Part model, mm, in its own coordinate system. A direction names the side the tool comes from. Round coordinates to 2 decimals unless told otherwise and drop trailing zeros. Write each loop counter-clockwise with the first axis right and the second up, starting at its lowest first coordinate (ties: lowest second). Pieces come first, ordered by that corner, then holes. Notation, with made-up numbers: M 81,-18 L 136,-18 A6 cw 136,-10 Z; hole C 22.5,3 d1. An arc over 180 degrees is marked long. Answer as a JSON object with one key per item and string values. Group by question number.
1. Drop flat-ended pins along their axis: pin 1 (2 mm diameter, centred on x = 13.4, z = 0, fed in from -Y); pin 2 (1.8 mm diameter, centred on x = -13, z = 1, fed in from +Y); pin 3 (3 mm diameter, centred on x = 0, z = 0, fed in from +Y); pin 4 (3 mm diameter, centred on x = 0, z = 0, fed in from -Y). Give the stop position or say it passes through.
2. Band-saw the part on C-C, the plane x = 1.5. Write the cut outline in (y, z).
3. Band-saw the part on B-B, the plane y = 3.55. Write the cut outline in (x, z).
4. Band-saw the part on A-A, the plane x = 9.8. Write the cut outline in (y, z), plus the area to 3 significant figures.
5. Drill centre lines: line 1 (X direction, y = 3.1, z = 0); line 2 (Y direction, x = 11.5, z = 1.25); line 3 (Z direction, x = 9.8, y = 0.5). Where is each one in solid material? Low to high. Write a range as from..to.
6. Two-plate mould, pull along Z, no slides. Class faces 1 (the face through (-8.628, 1.014, -2.473)), 2 (the face through (-5.15, 1.01, -0.03)), 3 (the face through (-8.75, 1.01, -0.03)), 4 (the face through (0, 0, -3)): +Z half, -Z half, draft (parallel to the pull), parting line (faces both ways), or undercut.
7. Which spindle directions (+Z, -Z, +X, -X, +Y, -Y) get a long thin tool onto all of the face, cutting with end or side? Do faces 5 (the face through (1, 1, 1)), 6 (the face through (1, 1.5, 1)), 7 (the face through (-12.685, 1.014, -0.225)). Say none if no direction does.
8. Band-saw the part on D-D, the plane x = 15.5. Write the cut outline in (y, z), plus the area to 3 significant figures.
from build123d import *

# Parameters (mm, degrees)
SKETCH1_W             = 3.5
SKETCH1_H             = 3.9
BOSS_EXTRUDE1_START   = -2
BOSS_EXTRUDE1_DEPTH   = 2
BOSS_EXTRUDE2_START   = -2
BOSS_EXTRUDE2_DEPTH   = 2
F_1_5MM_DOWEL_HOLE1_D = 1.5


with BuildPart() as part:
    # Sketch1 → Revolve1 (revolve)
    with BuildSketch(Plane.XY, mode=Mode.PRIVATE) as revolve1_sk:
        with Locations((1.75, 1.95)):
            Rectangle(SKETCH1_W, SKETCH1_H)
    revolve(revolve1_sk.sketch.rotate(Axis((0, 3.9, 0), (0, -1, 0)), 270), axis=Axis((0, 3.9, 0), (0, -1, 0)))

    # Sketch2 → Boss-Extrude1 (add)
    with BuildSketch(Plane.XZ.offset(BOSS_EXTRUDE1_START)):
        with BuildLine():
            Line((-1.868584713, 2.959457918), (-15.2, 2))
            ThreePointArc((-15.2, 2), (-17.2, 0), (-15.2, -2))
            Line((-15.2, -2), (-1.868584713, -2.959457918))
            ThreePointArc((-1.868584713, -2.959457918), (-3.5, 0), (-1.868584713, 2.959457918))
        make_face()
    extrude(amount=BOSS_EXTRUDE1_DEPTH)

    # Sketch3 → Boss-Extrude2 (add)
    with BuildSketch(Plane.XZ.offset(BOSS_EXTRUDE2_START)):
        with BuildLine():
            Line((1.868584713, -2.959457918), (15.2, -2))
            ThreePointArc((15.2, -2), (17.2, 0), (15.2, 2))
            Line((15.2, 2), (1.868584713, 2.959457918))
            ThreePointArc((1.868584713, 2.959457918), (3.5, 0), (1.868584713, -2.959457918))
        make_face()
    extrude(amount=BOSS_EXTRUDE2_DEPTH)

    # Sketch4 → Cut-Revolve1 (revolve, cut)
    with BuildSketch(Plane.XY, mode=Mode.PRIVATE) as cut_revolve1_sk:
        Polygon((2.45, 3.9), (0, 3.9), (0, 0), (2.35, 0), (2.35, 1), (1.2, 1), (1.2, 1.5), (2.45, 1.5), align=None)
    revolve(cut_revolve1_sk.sketch.rotate(Axis((0, 3.9, 0), (0, -1, 0)), 270), axis=Axis((0, 3.9, 0), (0, -1, 0)), mode=Mode.SUBTRACT)

    # Ø1.5mm Dowel Hole1 (through all)
    with Locations(Plane(origin=(0, 0, 0), x_dir=(-1, 0, 0), z_dir=(0, -1, 0))):
        with Locations((15.2, 0), (-15.2, 0), (13.4, 0), (11.6, 0), (9.8, 0), (8, 0), (6.2, 0), (4.4, 0), (-13.4, 0), (-11.6, 0), (-9.8, 0), (-8, 0), (-6.2, 0), (-4.4, 0)):
            Hole(F_1_5MM_DOWEL_HOLE1_D / 2)


solid = part.part
Worked answers:
{
 "1": {"pin 1": "stops at y = 0", "pin 2": "stops at y = 2", "pin 3": "stops at y = 1.5", "pin 4": "stops at y = 1"},
 "2": {"outline": "M 0,-3.16 L 3.9,-3.16 L 3.9,-1.94 L 1.5,-1.94 L 1.5,1.94 L 3.9,1.94 L 3.9,3.16 L 0,3.16 L 0,1.81 L 1,1.81 L 1,-1.81 L 0,-1.81 Z"},
 "3": {"outline": "C 0,0 d7; hole C 0,0 d4.9"},
 "4": {"outline": "M 0,-2.39 L 2,-2.39 L 2,-0.75 L 0,-0.75 Z; M 0,0.75 L 2,0.75 L 2,2.39 L 0,2.39 Z", "area": "6.55 mm^2"},
 "5": {"line 1": "x = -3.5..-2.45, 2.45..3.5", "line 2": "y = 0..2", "line 3": "z = -2.39..-0.75, 0.75..2.39"},
 "6": {"face 1": "-Z half", "face 2": "undercut", "face 3": "undercut", "face 4": "draft"},
 "7": {"face 5": "-Y", "face 6": "+Y", "face 7": "+Y, -Y"},
 "8": {"outline": "M 0,-1.98 L 2,-1.98 L 2,-0.69 L 0,-0.69 Z; M 0,0.69 L 2,0.69 L 2,1.98 L 0,1.98 Z", "area": "5.16 mm^2"}
}
